Could you check a few things on this drawing? It's one solid part, dimensions in mm from its lowest x, y, z. A direction names the side the tool comes from. Give positions to 0.01 mm unless a question says otherwise; leave off trailing zeros. Loops run counter-clockwise (first coordinate to the right, second up) from the corner with the lowest first, then second, coordinate; pieces in that order, holes last. Notation, with made-up numbers: (-30.5, 51.25) - (-0.5, 51.25) arc R23 ccw to (-0.5, 61.25) - close; hole circle Ø1 at (31.5, -23). An arc over 180 degrees is marked (long way). Write item = value, one per line.
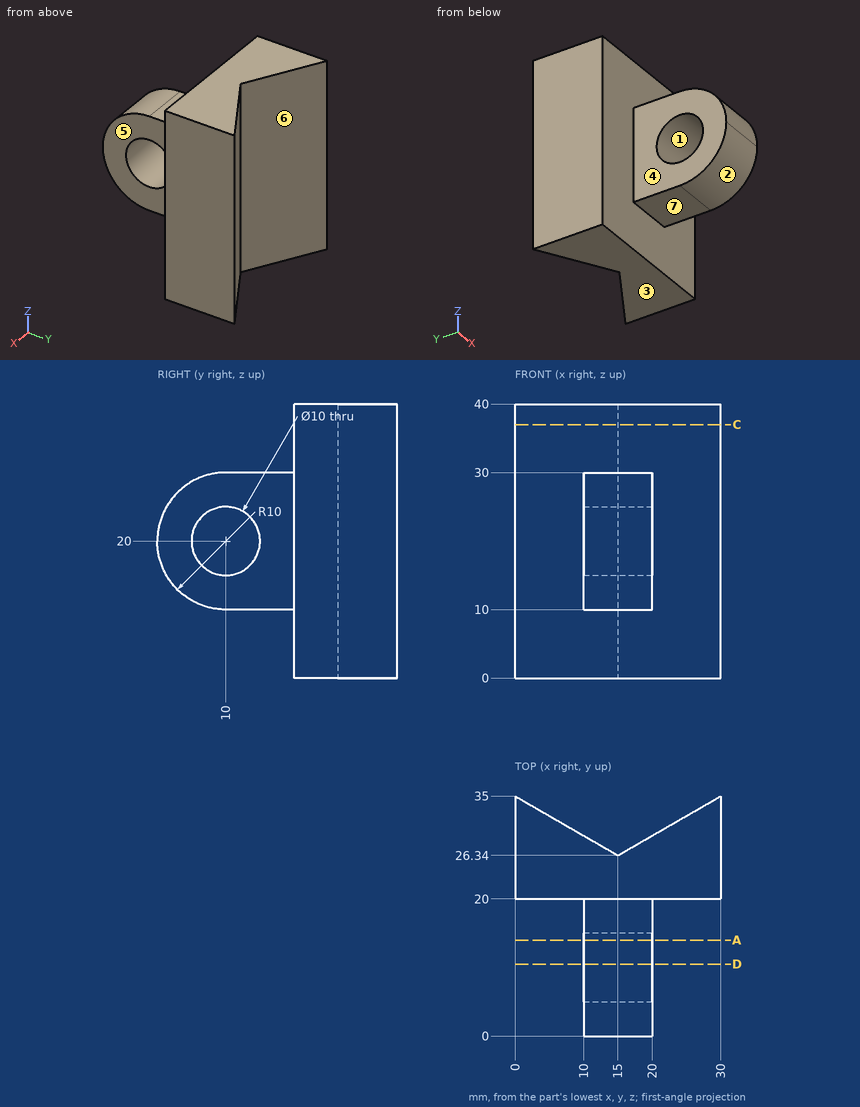
Q1. For pin 1 (3 mm diameter, centred on x = 21, z = 27, fed in from +Y); pin 2 (8 mm diameter, centred on x = 16, y = 14, fed in from -Z); pin 3 (6 mm diameter, centred on y = 13, z = 29, fed in from +X); pin 4 (6 mm diameter, centred on x = 5.5, y = 4, fed in from -Z), each with a flat end and sliding along its axis, tell me the tip position at first contact or that it passes through.
Output:
pin_1 = 30.67
pin_2 = 10
pin_3 = 20
pin_4 = through
Q2. We'd pull the mould along Y, two halves only. Please class the marked faces 1, 2 and 3: released by +Y, released by -Y, zero draft, split by the parting line, or undercut.
Output:
face_1 = undercut
face_2 = released by -Y
face_3 = zero draft
Q3. Imagine slicing it at C-C, the plane z = 37. Write out the boundary of the cut face in (x, y).
Output:
outline = (0, 20) - (30, 20) - (30, 35) - (15, 26.34) - (0, 35) - close
Q4. Imagine slicing it at D-D, the plane y = 10.5. Write out the boundary of the cut face in (x, z) (1 decimal).
Output:
outline = (10, 10) - (20, 10) - (20, 15) - (10, 15) - close; (10, 25) - (20, 25) - (20, 30) - (10, 30) - close
Q5. Which directions (+Z, -Z, +X, -X, +Y, -Y) give clear straight access to the entire face, cutting with the end or side of a thin tool? Please do the marked faces 4, 5, 6 and 7.
Output:
face_4 = +Z, -Z, -X, -Y
face_5 = +Z, -Z, +X, -Y
face_6 = +Z, -Z, +Y
face_7 = -Z, +X, -X, -Y
Q6. I need wall thicknesses on L1, parallel to Z at x = 13.75, y = 10; L2, parallel to X at y = 17.5, z = 13; L3, parallel to Z at x = 12, y = 5.5. Which ranges of each line are inside material? Lowest first, please.
Output:
L1 = 10 to 15, 25 to 30
L2 = 10 to 20
L3 = 11.07 to 17.82, 22.18 to 28.93
Q7. Imagine slicing it at A-A, the plane y = 14. Write out the boundary of the cut face in (x, z).
Output:
outline = (10, 10) - (20, 10) - (20, 17) - (10, 17) - close; (10, 23) - (20, 23) - (20, 30) - (10, 30) - close
